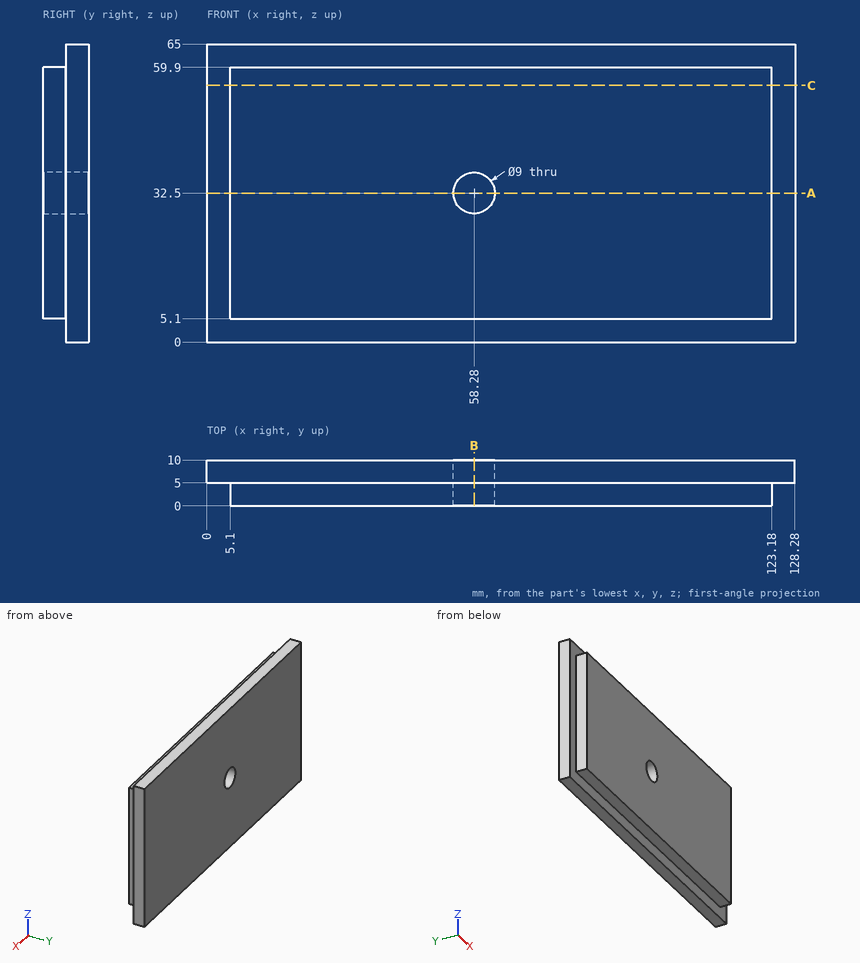
Could you check a few things on this drawing? It's one solid part, dimensions in mm from its lowest x, y, z. Coordinates: 2 decimals unless noted, no trailing zeros. Order: outer loops, then holes, each group sorted by start corner. A loop starts at its lowest first (then second) coordinate and runs counter-clockwise, first axis right, second up. Notation, with made-up numbers: (51.25, 32.5) -> (99.25, 32.5) arc R24 cw to (99.25, 42.5) -> close; hole circle Ø4 at (45, -36). An arc over 180 degrees is marked (long way). One line per item, written item: value. Start each with the question number.
1) Imagine slicing it at B-B on x = 58.28. List the corners of the cut face in (y, z) for me.
2) If I drill on L1, parallel to X at y = 4, z = 32.5; L2, parallel to Z at x = 77, y = 1; L3, parallel to X at y = 7.5, z = 32.5, over which ranges is the centre line in solid material (lowest first)? Write a range as [from, to].
3) Imagine slicing it at C-C on z = 56. List the corners of the cut face in (x, y) for me.
4) Imagine slicing it at A-A on z = 32.5. List the corners of the cut face in (x, y) for me, plus the area to 3 significant figures.
5) I'm going to push flat-ended pins straight in: pin 1 (2 mm diameter, centred on y = 2.5, z = 49.5, fed in from +X); pin 2 (4 mm diameter, centred on x = 91.5, y = 1.5, fed in from -Z); pin 3 (1.5 mm diameter, centred on y = 3, z = 30.5, fed in from -X); pin 4 (8 mm diameter, centred on x = 58.28, z = 32.5, fed in from -Y). Where does each tip first touch, or does it pass through?
Answer list:
1. outline: (0, 5.1) -> (5, 5.1) -> (5, 0) -> (10, 0) -> (10, 28) -> (0, 28) -> close; (0, 37) -> (10, 37) -> (10, 65) -> (5, 65) -> (5, 59.9) -> (0, 59.9) -> close
2. L1: x = [5.1, 53.78], [62.78, 123.18]
2. L2: z = [5.1, 59.9]
2. L3: x = [0, 53.78], [62.78, 128.28]
3. outline: (0, 5) -> (5.1, 5) -> (5.1, 0) -> (123.18, 0) -> (123.18, 5) -> (128.28, 5) -> (128.28, 10) -> (0, 10) -> close
4. outline: (0, 5) -> (5.1, 5) -> (5.1, 0) -> (53.78, 0) -> (53.78, 10) -> (0, 10) -> close; (62.78, 0) -> (123.18, 0) -> (123.18, 5) -> (128.28, 5) -> (128.28, 10) -> (62.78, 10) -> close
4. area: 1,140 mm2
5. pin 1: stops at x = 123.18
5. pin 2: stops at z = 5.1
5. pin 3: stops at x = 5.1
5. pin 4: passes through
